Part model, mm, in its own coordinate system. Coordinates: 2 decimals unless noted, no trailing zeros. Order: outer loops, then holes, each group sorted by start corner. A loop starts at its lowest first (then second) coordinate and runs counter-clockwise, first axis right, second up.
from build123d import *

# Parameters (mm, degrees)
SKETCH_W      = 17
SKETCH_H      = 110
PAD_DEPTH     = 6
SKETCH001_R   = 2.55
HOLE_DEPTH    = 6
SKETCH002_R   = 1.25
HOLE001_DEPTH = 6
CHAMFER_SIZE  = 2


with BuildPart() as part:
    # Sketch → Pad (new body)
    with BuildSketch(Plane.XY):
        Rectangle(SKETCH_W, SKETCH_H)
    extrude(amount=PAD_DEPTH)

    # Sketch001 → Hole (cut)
    with BuildSketch(Plane.XY):
        with Locations((0, 30)):
            Circle(SKETCH001_R)
        with Locations((0, -30)):
            Circle(SKETCH001_R)
    extrude(amount=HOLE_DEPTH, mode=Mode.SUBTRACT)

    # Sketch002 (on Face6 of Pad) → Hole001 (cut)
    with BuildSketch(Plane.XY.offset(6)):
        with Locations((0, 45)):
            Circle(SKETCH002_R)
        with Locations((0, -45)):
            Circle(SKETCH002_R)
        Circle(SKETCH002_R)
    extrude(amount=-HOLE001_DEPTH, mode=Mode.SUBTRACT)

    # Chamfer
    chamfer_edges = [part.edges().sort_by_distance(p)[0] for p in [
        (0, -55, 0),
        (0, 55, 0),
        (-8.5, 0, 0),
        (8.5, 0, 0),
    ]]
    chamfer(chamfer_edges, length=CHAMFER_SIZE)


solid = part.part
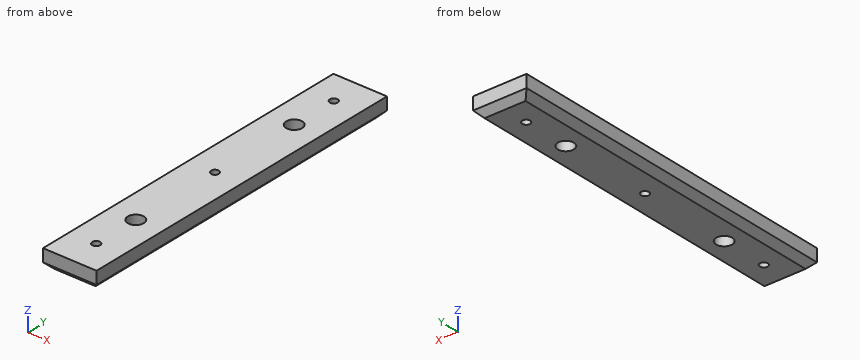
Q1. Cut at C-C on z = 4.8. Write the cut outline in (x, y).
Results list:
outline: (-8.5, -55) - (8.5, -55) - (8.5, 55) - (-8.5, 55) - close; hole circle Ø5.1 at (0, -30); hole circle Ø5.1 at (0, 30); hole circle Ø2.5 at (0, -45); hole circle Ø2.5 at (0, 0); hole circle Ø2.5 at (0, 45)
Q2. Cut at D-D on y = -30. Write the cut outline in (x, z).
Results list:
outline: (-8.5, 2) - (-6.5, 0) - (-2.55, 0) - (-2.55, 6) - (-8.5, 6) - close; (2.55, 0) - (6.5, 0) - (8.5, 2) - (8.5, 6) - (2.55, 6) - close
Q3. Cut at A-A on y = 0. Write the cut outline in (x, z).
Results list:
outline: (-8.5, 2) - (-6.5, 0) - (-1.25, 0) - (-1.25, 6) - (-8.5, 6) - close; (1.25, 0) - (6.5, 0) - (8.5, 2) - (8.5, 6) - (1.25, 6) - close
Q4. Pin check, flat tips, straight feed: pin 1 Ø3 at (x, y) = (0, 45) entering from +Z; pin 2 Ø1.5 at (x, z) = (-1.5, 1) entering from +Y. Stop position of each tip, or through.
Results list:
pin 1: stops at z = 6
pin 2: stops at y = 54.75
Q5. Cut at B-B on x = 0. Write the cut outline in (y, z).
Results list:
outline: (-55, 2) - (-53, 0) - (-46.25, 0) - (-46.25, 6) - (-55, 6) - close; (-43.75, 0) - (-32.55, 0) - (-32.55, 6) - (-43.75, 6) - close; (-27.45, 0) - (-1.25, 0) - (-1.25, 6) - (-27.45, 6) - close; (1.25, 0) - (27.45, 0) - (27.45, 6) - (1.25, 6) - close; (32.55, 0) - (43.75, 0) - (43.75, 6) - (32.55, 6) - close; (46.25, 0) - (53, 0) - (55, 2) - (55, 6) - (46.25, 6) - close
Q6. Wall check: line 1 along Y through (x, z) = (0, 2.8); line 2 along Y through (x, z) = (2, 5.6); line 3 along Y through (x, z) = (0.5, 2.7). Give the ranges that are in metal, low to high.
Results list:
line 1: y = -55 to -46.25, -43.75 to -32.55, -27.45 to -1.25, 1.25 to 27.45, 32.55 to 43.75, 46.25 to 55
line 2: y = -55 to -31.58, -28.42 to 28.42, 31.58 to 55
line 3: y = -55 to -46.15, -43.85 to -32.5, -27.5 to -1.15, 1.15 to 27.5, 32.5 to 43.85, 46.15 to 55
